Verification items for the finished model (mm, model axes). A direction names the side the tool comes from. Round coordinates to 2 decimals unless told otherwise and drop trailing zeros. Write each loop counter-clockwise with the first axis right and the second up, starting at its lowest first coordinate (ties: lowest second). Pieces come first, ordered by that corner, then holes. Notation, with made-up numbers: (36, 64) - (56, 64) arc R17 ccw to (56, 94) - close; hole circle Ø8 at (79, 6). An arc over 180 degrees is marked (long way). Answer as a JSON object with one key per item and string values.
Autodesk Inventor part; units mm, degrees
ref_plane "1_XY" through (3, 0, 0) normal (1, 0, 0) x (0, 0, -1)
ref_plane "1_YZ" through (3, 0, 0) normal (0, 0, -1) x (0, 1, 0)
ref_plane "1_ZX" through (3, 0, 0) normal (0, 1, 0) x (1, 0, 0)
sketch "Sketch_6" plane through (0, 0, 0) normal (0, 0, 1) x (1, 0, 0)
  line L0 (6, 0) -> (0, 0)
  line L1 (0, 6.05) -> (0, 5.3)
  arc A0 (0, 5.3) -> (0.3, 5) centre (0.3, 5.3) ccw
  line L2 (0.3, 5) -> (5.7, 5)
  arc A1 (5.7, 5) -> (6, 5.3) centre (5.7, 5.3) ccw
  line L3 (6, 5.3) -> (6, 6.05)
  arc A2 (6, 6.05) -> (5.85, 6.2) centre (5.85, 6.05) ccw
  line L4 (5.85, 6.2) -> (4.8, 6.2)
  line L5 (4.8, 6.2) -> (4.8, 6.73)
  line L6 (4.8, 6.73) -> (3.9525, 6.73)
  arc A3 (2.0475, 6.73) -> (3.9525, 6.73) centre (3, 8) ccw
  line L7 (2.0475, 6.73) -> (1.2, 6.73)
  line L8 (1.2, 6.73) -> (1.2, 6.2)
  line L9 (1.2, 6.2) -> (0.15, 6.2)
  arc A4 (0.15, 6.2) -> (0, 6.05) centre (0.15, 6.05) ccw
revolve "Revolution1" add sketch "Sketch_6" angle 360 about axis through (6, 0, 0) along (1, 0, 0)
ref_plane "1_XY" through (3, 0, 0) normal (1, 0, 0) x (0, 0, -1)
ref_plane "1_YZ" through (3, 0, 0) normal (0, 0, -1) x (0, 1, 0)
ref_plane "1_ZX" through (3, 0, 0) normal (0, 1, 0) x (1, 0, 0)
ref_plane "Dummy_XY" through (0, 0, 0) normal (1, 0, 0) x (0, 0, -1)
ref_plane "Dummy_YZ" through (0, 0, 0) normal (0, 0, -1) x (0, 1, 0)
ref_plane "Dummy_ZX" through (0, 0, 0) normal (0, 1, 0) x (1, 0, 0)
ref_plane "shield1_XY" through (0.4, 0, 0) normal (1, 0, 0) x (0, 0, -1)
ref_plane "shield1_YZ" through (0.4, 0, 0) normal (0, 0, -1) x (0, 1, 0)
ref_plane "shield1_ZX" through (0.4, 0, 0) normal (0, 1, 0) x (1, 0, 0)
ref_plane "shield2_XY" through (5.6, 0, 0) normal (-1, 0, 0) x (0, 0, -1)
ref_plane "shield2_YZ" through (5.6, 0, 0) normal (0, 0, -1) x (0, -1, 0)
ref_plane "shield2_ZX" through (5.6, 0, 0) normal (0, -1, 0) x (-1, 0, 0)
properties part number "RF-2210X2HH_ir"
Q1. Set-up check for faces 4 (the flat face through (1.2, 4.5, -4.5)), 5 (the flat face through (6, 4, -4)), 6 (the cylindrical face through (5.32, 2.86, 5.5)): record each of +Z, -Z, +X, -X, +Y, -Y from which the full face is reachable in a straight line by a thin tool's end or side.
Geometry check:
{"face 4": "-X", "face 5": "+Z, -Z, +X, +Y, -Y", "face 6": "+X"}
Q2. Release check for a two-part mould opening along Y. For faces 1 (the cylindrical face through (3.04, -1.08, -4.88)), 2 (the cylindrical face through (1.62, -1.46, 6.57)), 3 (the flat face through (4.8, 4.5, -4.5)) record: released by +Y, released by -Y, zero draft, split by the parting line, or undercut.
Geometry check:
{"face 1": "undercut", "face 2": "split by the parting line", "face 3": "zero draft"}
Q3. Section check C-C, the plane x = 3.05. Record the cut outline in (y, z).
Geometry check:
{"outline": "circle Ø12.83 at (0, 0); hole circle Ø10 at (0, 0)"}
Q4. Material ranges on line 1 along Z through (x, y) = (4.3, 0); line 2 along Z through (x, y) = (3.35, 0); line 3 along Y through (x, z) = (0.9, -4), recorded low to high. Write a range as [from, to].
Geometry check:
{"line 1": "z = [-6.73, -5], [5, 6.73]", "line 2": "z = [-6.45, -5], [5, 6.45]", "line 3": "y = [-4.74, -3], [3, 4.74]"}
Q5. Gauge pin test, flat end, axial feed: P1, Ø1, axis at x = 2.5, z = 4.5, coming from the -Y side. Record the tip position at first contact, or that the pin passes through.
Geometry check:
{"P1": "stops at y = -5.21"}
